Could you check a few things on this model? Use its own coordinates, in mm. A direction names the side the tool comes from. Coordinates: 2 decimals unless noted, no trailing zeros. Loops run counter-clockwise (first coordinate to the right, second up) from the corner with the lowest first, then second, coordinate; pieces in that order, holes last. Notation, with made-up numbers: M -26,-6 L 3,-6 A20 ccw 3,7 Z; hole C -3.75,18 d2. An arc over 180 degrees is marked long. Write each question's results on one line, items separated by ' | '.
```python
from build123d import *

# Parameters (mm, degrees)
SKETCH_1_W             = 200
SKETCH_1_H             = 150
EXTRUDE_1_DEPTH        = 1
EXTRUDE_2_DEPTH        = 200
PATTERN_LINEAR_1_COUNT = 5
PATTERN_LINEAR_1_PITCH = 20
SKETCH_5_W             = 178
SKETCH_5_H             = 10
CUT_EXTRUDE_1_DEPTH    = 1
PATTERN_LINEAR_2_COUNT = 5
PATTERN_LINEAR_2_PITCH = 20


with BuildPart() as part:
    # 草图1 → 凸台-拉伸1 (new body)
    with BuildSketch(Plane(origin=(0, 0, 0), x_dir=(1, 0, 0), z_dir=(0, 1, 0))):
        with Locations((100, -75)):
            Rectangle(SKETCH_1_W, SKETCH_1_H)
    extrude(amount=EXTRUDE_1_DEPTH)

    # 草图4 → 凸台-拉伸2 (add)
    with BuildSketch(Plane.ZY):
        Polygon((8, 1), (10, 1), (20.467293485, 7.043294711), (19.967293485, 7.909320115), align=None)
    extrude_2 = extrude(amount=-EXTRUDE_2_DEPTH)

    # 阵列(线性)1: 凸台-拉伸2 ×5
    with Locations(*[(0, 0, i * PATTERN_LINEAR_1_PITCH) for i in range(1, PATTERN_LINEAR_1_COUNT)]):
        add(extrude_2)

    # 草图5 → 切除-拉伸1 (cut)
    with BuildSketch(Plane(origin=(0, 1, 0), x_dir=(1, 0, 0), z_dir=(0, 1, 0))):
        with Locations((99, -15)):
            Rectangle(SKETCH_5_W, SKETCH_5_H)
    cut_extrude_1 = extrude(amount=-CUT_EXTRUDE_1_DEPTH, mode=Mode.SUBTRACT)

    # 阵列(线性)2: 切除-拉伸1 ×5
    with Locations(*[(0, 0, i * PATTERN_LINEAR_2_PITCH) for i in range(1, PATTERN_LINEAR_2_COUNT)]):
        add(cut_extrude_1, mode=Mode.SUBTRACT)


solid = part.part
```
(1) Please list where these lines run through material, in increasing order: probe 1 along Z at (x, y) = (10.5, 0.5); probe 2 along Z at (x, y) = (128.5, 2.75); probe 3 along Z at (x, y) = (110, 7.5). Write a range as from..to.
Reported:
probe 1: z = 0..10, 20..30, 40..50, 60..70, 80..90, 100..150 | probe 2: z = 11.03..13.03, 31.03..33.03, 51.03..53.03, 71.03..73.03, 91.03..93.03 | probe 3: z = 19.26..20.2, 39.26..40.2, 59.26..60.2, 79.26..80.2, 99.26..100.2
(2) Imagine slicing it at D-D, the plane z = 134.5. List the corners of the cut face in (x, y) for me, and give its area (3 significant figures).
Reported:
outline: M 0,0 L 200,0 L 200,1 L 0,1 Z | area: 200 mm2
(3) Imagine slicing it at A-A, the plane y = 5.75. List the corners of the cut face in (x, z) for me.
Reported:
outline: M 0,16.23 L 200,16.23 L 200,18.23 L 0,18.23 Z; M 0,36.23 L 200,36.23 L 200,38.23 L 0,38.23 Z; M 0,56.23 L 200,56.23 L 200,58.23 L 0,58.23 Z; M 0,76.23 L 200,76.23 L 200,78.23 L 0,78.23 Z; M 0,96.23 L 200,96.23 L 200,98.23 L 0,98.23 Z
(4) If we mould it in two halves opening along Y, with no side actions, what happens to faces 3 (the flat face through (0, 1.3, 69.8)), 4 (the flat face through (99, 1, 23)), 5 (the flat face through (98.6, 4.503, 54.067))? For each: released by +Y, released by -Y, zero draft, split by the parting line, or undercut.
Reported:
face 3: zero draft | face 4: undercut | face 5: released by +Y
(5) Imagine slicing it at B-B, the plane x = 161.5. State how many separate pieces and enclosed holes the cut face has, and give its area (3 significant figures).
Reported:
separate pieces: 6 | enclosed holes: 0 | area: 165 mm2
(6) Will this pin go through, and if not, where does the flat tip stop? P1, Ø9, axis at x = 84, z = 2.5, coming from the +Y side.
Reported:
P1: stops at y = 1
(7) Imagine slicing it at C-C, the plane z = 55. List the corners of the cut face in (x, y) for me, and give its area (3 significant figures).
Reported:
outline: M 0,0 L 10,0 L 10,1 L 0,1 Z; M 0,3.89 L 200,3.89 L 200,5.04 L 0,5.04 Z; M 188,0 L 200,0 L 200,1 L 188,1 Z | area: 253 mm2
(8) Which directions (+Z, -Z, +X, -X, +Y, -Y) give clear straight access to the entire face, cutting with the end or side of a thin tool? Please do faces 1 (the flat face through (98.6, 4.503, 34.067)), 2 (the flat face through (200, 1.3, 69.8)).
Reported:
face 1: +X, -X, +Y | face 2: +Z, -Z, +X, +Y, -Y
